from build123d import *

# Parameters (mm, degrees)
SKETCH_1_R          = 26.5
EXTRUDE_1_DEPTH     = 5.5
CHAMFER_1_SIZE      = 0.5
SKETCH_4_R          = 2
CUT_EXTRUDE_2_DEPTH = 38.878093933
CHAMFER_2_SIZE      = 1
SKETCH_5_R          = 1.5
CUT_EXTRUDE_3_DEPTH = 38.878093933
CUT_EXTRUDE_4_DEPTH = 3


with BuildPart() as part:
    # Эскиз1 → Бобышка-Вытянуть1 (new body)
    with BuildSketch(Plane(origin=(0, 0, 0), x_dir=(1, 0, 0), z_dir=(0, 1, 0))):
        with Locations(Location((0, 0, 0), (0, 0, 270))):
            Circle(SKETCH_1_R)
    extrude(amount=EXTRUDE_1_DEPTH)

    # Фаска1
    chamfer_1_edges = [part.edges().sort_by_distance(p)[0] for p in [
        (0, 5.5, -26.5),
    ]]
    chamfer(chamfer_1_edges, length=CHAMFER_1_SIZE)

    # Эскиз4 → Вырез-Вытянуть2 (cut, through all)
    with BuildSketch(Plane(origin=(0, 5.5, 0), x_dir=(1, 0, 0), z_dir=(0, 1, 0))):
        with Locations(Location((-15.556349186, 15.556349186, 0), (0, 0, 270))):
            Circle(SKETCH_4_R)
        with Locations(Location((15.556349186, 15.556349186, 0), (0, 0, 270))):
            Circle(SKETCH_4_R)
        with Locations(Location((15.556349186, -15.556349186, 0), (0, 0, 270))):
            Circle(SKETCH_4_R)
        with Locations(Location((-15.556349186, -15.556349186, 0), (0, 0, 270))):
            Circle(SKETCH_4_R)
    extrude(amount=-CUT_EXTRUDE_2_DEPTH, mode=Mode.SUBTRACT)

    # Фаска2
    chamfer_2_edges = [part.edges().sort_by_distance(p)[0] for p in [
        (-15.556349186, 5.5, 13.556349186),
        (15.556349186, 5.5, 13.556349186),
        (15.556349186, 5.5, -17.556349186),
        (-15.556349186, 5.5, -17.556349186),
    ]]
    chamfer(chamfer_2_edges, length=CHAMFER_2_SIZE)

    # Эскиз5 → Вырез-Вытянуть3 (cut, through all)
    with BuildSketch(Plane(origin=(0, 5.5, 0), x_dir=(1, 0, 0), z_dir=(0, 1, 0))):
        with Locations(Location((0, 12.5, 0), (0, 0, 270))):
            Circle(SKETCH_5_R)
        with Locations(Location((12.5, 0, 0), (0, 0, 270))):
            Circle(SKETCH_5_R)
        with Locations(Location((0, -12.5, 0), (0, 0, 270))):
            Circle(SKETCH_5_R)
        with Locations(Location((-12.5, 0, 0), (0, 0, 270))):
            Circle(SKETCH_5_R)
        with Locations(Location((10.606601718, 10.606601718, 0), (0, 0, 270))):
            Circle(SKETCH_5_R)
        with Locations(Location((10.606601718, -10.606601718, 0), (0, 0, 270))):
            Circle(SKETCH_5_R)
        with Locations(Location((-10.606601718, -10.606601718, 0), (0, 0, 270))):
            Circle(SKETCH_5_R)
        with Locations(Location((-10.606601718, 10.606601718, 0), (0, 0, 270))):
            Circle(SKETCH_5_R)
    extrude(amount=-CUT_EXTRUDE_3_DEPTH, mode=Mode.SUBTRACT)

    # Эскиз6 → Вырез-Вытянуть4 (cut)
    with BuildSketch(Plane.XZ):
        with BuildLine():
            Line((6.5, 6.92820323), (6.5, 25.690465157))
            ThreePointArc((6.5, 25.690465157), (0, 26.5), (-6.5, 25.690465157))
            Line((-6.5, 25.690465157), (-6.5, 6.92820323))
            ThreePointArc((-6.5, 6.92820323), (0, -9.5), (6.5, 6.92820323))
        make_face()
    extrude(amount=-CUT_EXTRUDE_4_DEPTH, mode=Mode.SUBTRACT)


solid = part.part
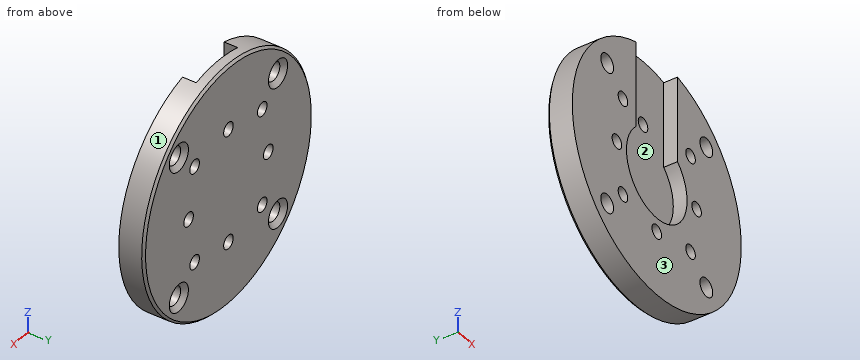
Source: CAD feature listing. Evaluate the final solid. Frame: model axes, mm. Face numbers are marked on the shaded views. Give positions to 0.01 mm unless a question says otherwise; leave off trailing zeros. Write each loop counter-clockwise with the first axis right and the second up, starting at its lowest first coordinate (ties: lowest second). Pieces come first, ordered by that corner, then holes. Notation, with made-up numbers: (58.25, 84) -> (99.25, 84) arc R25 ccw to (99.25, 106) -> close; hole circle Ø11 at (-23.5, 85.5). An arc over 180 degrees is marked (long way). Write item = value, one per line.
Q1. Mould query, pull axis X, two halves, no side actions, for the marked faces 1, 2 and 3. Classes: +X half, -X half, draft (parallel to the pull), parting line (faces both ways), or undercut.
Here are the results:
face_1 = parting line
face_2 = undercut
face_3 = draft
Q2. Cut plane B-B on y = 0.8. State how many separate pieces and enclosed holes the cut face has, then the cut area to 3 significant figures.
Here are the results:
separate_pieces = 1
enclosed_holes = 11
area = 1,590 mm²
Q3. First-contact query: pin 1 (1.5 mm diameter, centred on y = 1.5, z = 13, fed in from +X); pin 2 (2.5 mm diameter, centred on y = 2, z = 20, fed in from -X); pin 3 (3 mm diameter, centred on y = 3.5, z = 16.5, fed in from -X). Flat tips, straight axial feed; report the tip coordinate or a pass-through.
Here are the results:
pin_1 = 23.5
pin_2 = -18.73
pin_3 = -21.85
Q4. Cut plane A-A on x = 0. Return loops of the section in (y, z).
Here are the results:
outline = (0, -26.5) -> (5, -26.5) -> (5.5, -26) -> (5.5, -14) -> (0, -14) -> close; (0, -11) -> (5.5, -11) -> (5.5, 11) -> (3, 11) -> (3, -9.5) -> (0, -9.5) -> close; (3, 14) -> (5.5, 14) -> (5.5, 26) -> (5, 26.5) -> (3, 26.5) -> close
Q5. Line query: line 1 (Z direction, x = -17, y = 2.6); line 2 (X direction, y = 2.95, z = 1); line 3 (X direction, y = 1.95, z = 22.5). Output: solid intervals per line, ascending. Write a range as from..to.
Here are the results:
line_1 = -20.33..-16.94, -14.17..14.17, 16.94..20.33
line_2 = -26.48..-13.62, -11.38..-9.45, 9.45..11.38, 13.62..26.48
line_3 = -14..-6.5, 6.5..14
